Autodesk Inventor part; units mm, degrees
ref_plane "YZ Plane" through (0, 0, 0) normal (1, 0, 0) x (0, 1, 0)
ref_plane "XZ Plane" through (0, 0, 0) normal (0, 1, 0) x (-1, 0, 0)
ref_plane "XY Plane" through (0, 0, 0) normal (0, 0, 1) x (1, 0, 0)
sketch "Sketch1" plane through (0, 0, 0) normal (0, 0, 1) x (1, 0, 0)
  line L0 (-46.5, 0) -> (-46.5, -16.75)
  line L1 (-46.5, -16.75) -> (-43.5, -16.75)
  arc A0 (-4.25, -68) -> (-43.5, -26.7985) centre (-45.5, -68) ccw
  line L2 (-43.5, -16.75) -> (-43.5, -26.7985)
  line L3 (-4.5, 0) -> (-4.5, -43)
  line L4 (-4.5, -43) -> (0, -43)
  line L5 (-20, 0) -> (-20, 3)
  line L6 (-20, 3) -> (-30, 3)
  line L7 (-30, 3) -> (-30, 0)
  line L8 (-46.5, 0) -> (-30, 0)
  line L9 (-20, 0) -> (-4.5, 0)
  line L10 (-38.5, -17.5464) -> (-38.5, -7)
  line L11 (-36.5, -5) -> (-11.5, -5)
  line L12 (-9.5, -7) -> (-9.5, -29.6521)
  arc A1 (-12.8268, -31.1486) -> (-36.8512, -19.5154) centre (-45.5, -68) ccw
  arc A2 (-38.5, -17.5464) -> (-36.8512, -19.5154) centre (-36.5, -17.5464) ccw
  arc A3 (-36.5, -5) -> (-38.5, -7) centre (-36.5, -7) ccw
  arc A4 (-9.5, -7) -> (-11.5, -5) centre (-11.5, -7) ccw
  arc A5 (-12.8268, -31.1486) -> (-9.5, -29.6521) centre (-11.5, -29.6521) ccw
  line L13 (-4.25, -68) -> (0, -68)
  line L14 (46.5, 0) -> (46.5, -16.75)
  line L15 (46.5, -16.75) -> (43.5, -16.75)
  arc A6 (43.5, -26.7985) -> (4.25, -68) centre (45.5, -68) ccw
  line L16 (43.5, -16.75) -> (43.5, -26.7985)
  line L17 (4.5, 0) -> (4.5, -43)
  line L18 (4.5, -43) -> (0, -43)
  line L19 (20, 0) -> (20, 3)
  line L20 (20, 3) -> (30, 3)
  line L21 (30, 3) -> (30, 0)
  line L22 (46.5, 0) -> (30, 0)
  line L23 (20, 0) -> (4.5, 0)
  line L24 (38.5, -17.5464) -> (38.5, -7)
  line L25 (36.5, -5) -> (11.5, -5)
  line L26 (9.5, -7) -> (9.5, -29.6521)
  arc A7 (36.8512, -19.5154) -> (12.8268, -31.1486) centre (45.5, -68) ccw
  arc A8 (36.8512, -19.5154) -> (38.5, -17.5464) centre (36.5, -17.5464) ccw
  arc A9 (38.5, -7) -> (36.5, -5) centre (36.5, -7) ccw
  arc A10 (11.5, -5) -> (9.5, -7) centre (11.5, -7) ccw
  arc A11 (9.5, -29.6521) -> (12.8268, -31.1486) centre (11.5, -29.6521) ccw
  line L27 (4.25, -68) -> (0, -68)
  point P0 (0, 0)
  point P1 (-9.5, -34.391)
  point P2 (-38.5, -19.25)
  point P3 (9.5, -34.391)
  point P4 (38.5, -19.25)
  dimension "d1" = 46.5
  dimension "d3" = 3
  dimension "d5" = 82.5
  dimension "d7" = 45.5
  dimension "d10" = 10
  dimension "d24" = 10
  dimension "d25" = 20
  dimension "d32" = 8
  dimension "d33" = 5
  dimension "d36" = 15.5
  dimension "d37" = 16.5
  dimension "d38" = 16.75
  dimension "d39" = 5
  dimension "d40" = 2
  dimension "d45" = 8
  dimension "d49" = 68
  dimension "d50" = 25
extrude "Extrusion6" add sketch "Sketch1" along normal blind 3
properties part number "OpenROV 2_3 Dev Ducting Brace"
Model file for the job. Use its own axes, mm. A direction names the side the tool comes from. Round coordinates to 2 decimals unless told otherwise and drop trailing zeros. Write each loop counter-clockwise with the first axis right and the second up, starting at its lowest first coordinate (ties: lowest second). Pieces come first, ordered by that corner, then holes. Notation, with made-up numbers: (-8.75, -4) - (28.25, -4) arc R25 cw to (28.25, 8) - close; hole circle Ø6 at (12, -35.5). An arc over 180 degrees is marked (long way). One line per item, written item: value.
(1) Drop flat-ended pins along their axis: P1, Ø1.5, axis at x = 1.5, z = 2, coming from the +Y side; P2, Ø0.9, axis at y = 2, z = 1.5, coming from the -X side; P3, Ø1.5, axis at y = -18.5, z = 1.5, coming from the +X side. Give the stop position or say it passes through.
Values follow:
P1: stops at y = -43
P2: stops at x = -30
P3: stops at x = 43.5
(2) Cut at A-A, the plane y = -18.5. Give the cut face in (x, z), plus the area to 3 significant figures.
Values follow:
outline: (-43.5, 0) - (-38.26, 0) - (-38.26, 3) - (-43.5, 3) - close; (-9.5, 0) - (-4.5, 0) - (-4.5, 3) - (-9.5, 3) - close; (4.5, 0) - (9.5, 0) - (9.5, 3) - (4.5, 3) - close; (38.26, 0) - (43.5, 0) - (43.5, 3) - (38.26, 3) - close
area: 61.5 mm²
(3) Two-plate mould, pull along X, no slides. Class faces 1 (the flat face through (-45, -16.75, 1)), 2 (the cylindrical face through (-38.021, -18.845, 1.479)), 3 (the flat face through (12, 0, 1)), 4 (the flat face through (-30, 2, 1)): pulls with the +X half, pulls with the -X half, needs draft (parallel to the pull), parting line crosses it, or undercut.
Values follow:
face 1: needs draft
face 2: undercut
face 3: undercut
face 4: pulls with the -X half
(4) Cut at B-B, the plane x = 22. Give the cut face in (y, z), plus the area to 3 significant figures.
Values follow:
outline: (-34.1, 0) - (-24.72, 0) - (-24.72, 3) - (-34.1, 3) - close; (-5, 0) - (3, 0) - (3, 3) - (-5, 3) - close
area: 52.1 mm²
(5) Cut at D-D, the plane z = 2.35. Give the number of separate pieces and of enclosed holes in the cut face, plus the area to 3 significant figures.
Values follow:
separate pieces: 1
enclosed holes: 2
area: 2,050 mm²
(6) Cut at C-C, the plane y = -33.5. Give the cut face in (x, z).
Values follow:
outline: (-22.89, 0) - (-4.5, 0) - (-4.5, 3) - (-22.89, 3) - close; (4.5, 0) - (22.89, 0) - (22.89, 3) - (4.5, 3) - close
(7) 3-axis set-ups, long thin cutter, end or side, ignore diameter. For faces 5 (the flat face through (45, -16.75, 1)), 6 (the flat face through (38, 0, 1)), 7 (the flat face through (-43.5, -22, 1)), 8 (the cylindrical face through (-37.93, -5.6, 1.48)): which of +Z, -Z, +X, -X, +Y, -Y reach the whole face in a straight line?
Values follow:
face 5: +Z, -Z, +X, -Y
face 6: +Z, -Z, +X, +Y
face 7: +Z, -Z, -X, -Y
face 8: +Z, -Z
(8) Wall check: probe 1 along X at (y, z) = (-16, 0.5); probe 2 along X at (y, z) = (-25, 0.3); probe 3 along X at (y, z) = (-1.5, 1.75). Give the ranges that are in metal, low to high.
Values follow:
probe 1: x = -46.5 to -38.5, -9.5 to -4.5, 4.5 to 9.5, 38.5 to 46.5
probe 2: x = -43.5 to -21.49, -9.5 to -4.5, 4.5 to 9.5, 21.49 to 43.5
probe 3: x = -46.5 to -4.5, 4.5 to 46.5
